Check sheet for the modelled part. Datum: model origin and axes. Units: mm. Face numbers are marked on the shaded views. A direction names the side the tool comes from. Round coordinates to 2 decimals unless told otherwise and drop trailing zeros. Order: outer loops, then holes, each group sorted by start corner. A loop starts at its lowest first (then second) coordinate and runs counter-clockwise, first axis right, second up.
(1) Depth check by flat-ended pin: pin 1 (2 mm diameter, centred on x = 0.5, y = 15.5, fed in from -Z); pin 2 (2 mm diameter, centred on y = 14, z = -48.5, fed in from +X); pin 3 (8 mm diameter, centred on x = 8.5, z = -13, fed in from +Y). Enter the tip coordinate at first touch or a pass-through.
(2) Mould release check, pull along X, two halves, no side actions. Record for the marked faces 3, 4, 5 and 6: released by +X, released by -X, zero draft, split by the parting line, or undercut.
(3) Sectioned sample at A-A, the plane x = 46.5. Enter the section's corners in (y, z).
(4) Sectioned sample at B-B, the plane y = 18.5. Enter the section's corners in (x, z).
(5) Tool access check on the marked faces 1 and 2. Record the directions out of +Z, -Z, +X, -X, +Y, -Y that give a thin tool (end or side, any length) a straight path to the whole face; none if there is none.
(6) Thickness scan on probe 1 along Z at (x, y) = (55, 10.25); probe 2 along X at (y, z) = (17.25, -13); probe 3 along X at (y, z) = (1, -40.5). Record the ranges inside material, lowest first.
(7) Sectioned sample at C-C, the plane z = -11. Enter the section's corners in (x, y).
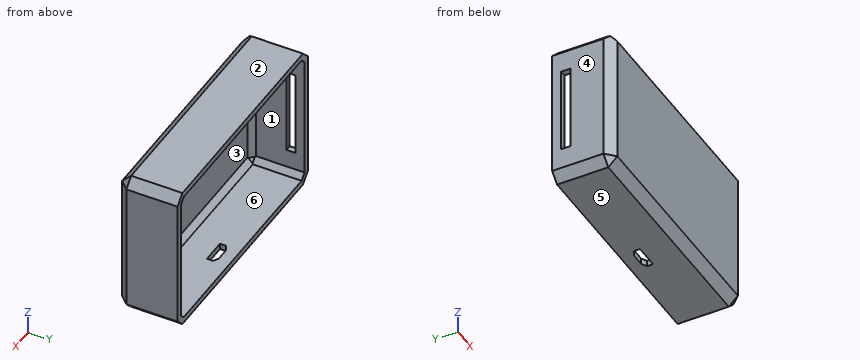
Autodesk Inventor part; units mm, degrees
ref_plane "YZ Plane" through (0, 0, 0) normal (1, 0, 0) x (0, 1, 0)
ref_plane "XZ Plane" through (0, 0, 0) normal (0, 1, 0) x (-1, 0, 0)
ref_plane "XY Plane" through (0, 0, 0) normal (0, 0, 1) x (1, 0, 0)
sketch "Náčrt1" plane through (0, 0, 0) normal (0, 1, 0) x (-1, 0, 0)
  line L0 (0, 0) -> (-80, 0)
  line L1 (-80, 0) -> (-80, -49)
  line L2 (-80, -49) -> (0, -49)
  line L3 (0, -49) -> (0, 0)
  dimension "d0" = 80
  dimension "d1" = 49
extrude "Vysunutí1" add sketch "Náčrt1" along normal blind 20
chamfer "Zkosení1" distance 3 angle 45 7 edges at (80, 10, 0) (40, 0, 0) (0, 0, -24.5) (0, 10, -49) (80, 10, -49) (40, 0, -49) (80, 0, -24.5)
chamfer "Zkosení2" distance 3 angle 45 1 edges at (0, 11.5, 0)
shell "Skořepina1" thickness 2 removed faces 1 at (27.6667, 20, -32.6667)
sketch "Náčrt2" plane through (0, 3, -46) normal (-1, 0, 0) x (0, 0, 1)
  line L0 (7, 14) -> (36, 14)
  line L1 (36, 14) -> (36, 11)
  line L2 (36, 11) -> (7, 11)
  line L3 (7, 11) -> (7, 14)
  line L4 (0, 0) -> (0, 17)
  line L5 (0, -3) -> (43, -3)
  line L6 (43, 0) -> (0, 0)
  line L7 (0, 17) -> (43, 17)
  point P0 (46, -3)
  dimension "d11" = 29
  dimension "d12" = 3
  dimension "d13" = 7
  dimension "d17" = 3
extrude "Vysunutí2" cut sketch "Náčrt2" against normal blind 2.5
sketch "Náčrt3" plane through (0, 14, -39) normal (0, 0, 1) x (1, 0, 0)
  point P0 (0, -14)
sketch "Náčrt4" plane through (77, 3, -49) normal (0, 0, -1) x (-1, 0, 0)
  line L0 (28, 13) -> (36, 13)
  line L1 (36, 13) -> (36, 10)
  line L2 (36, 10) -> (28, 10)
  line L3 (28, 10) -> (28, 13)
  line L4 (0, 0) -> (0, 17)
  line L5 (74, 0) -> (0, 0)
  line L6 (0, 17) -> (74, 17)
  point P0 (77, -3)
  dimension "d20" = 8
  dimension "d21" = 3
  dimension "d22" = 28
  dimension "d39" = 4
extrude "Vysunutí3" cut sketch "Náčrt4" against normal blind 2.5
chamfer "Zkosení3" distance 1 angle 60 1 edges at (49, 16, -48) measured on face at (49, 14, -48.3333)
chamfer "Zkosení4" distance 1 angle 60 1 edges at (41, 16, -48) measured on face at (41, 15, -48.3333)
sketch "Náčrt5" plane through (77, 3, 0) normal (0, 0, 1) x (1, 0, 0)
  point P0 (-77, -3)
sketch "Náčrt6" plane through (77, 3, -49) normal (0, 0, -1) x (-1, 0, 0)
  point P0 (77, -3)
sketch "Náčrt7" plane through (2, 3.8284, -3.8284) normal (1, 0, 0) x (0, 0, -1)
  point P0 (-3.8284, -3.8284)
properties part number "Base"
Derived:
1. pin 1: stops at z = -47.5
1. pin 2: stops at x = 78.5
1. pin 3: stops at y = 2
2. face 3: undercut
2. face 4: released by -X
2. face 5: zero draft
2. face 6: undercut
3. outline: (0, -46) - (3, -49) - (13, -49) - (13, -47) - (3.83, -47) - (2, -45.17) - (2, -3.83) - (3.83, -2) - (20, -2) - (20, 0) - (3, 0) - (0, -3) - close; (16, -49) - (20, -49) - (20, -47) - (16, -47) - close
4. outline: (0, -46) - (3, -49) - (77, -49) - (80, -46) - (80, -3) - (77, 0) - (3, 0) - (0, -3) - close; hole (2, -45.17) - (3.83, -47) - (76.17, -47) - (78, -45.17) - (78, -3.83) - (76.17, -2) - (3.83, -2) - (2, -3.83) - close
5. face 1: +Y
5. face 2: +Z, +X, -X, +Y, -Y
6. probe 1: z = -49 to -47, -2 to 0
6. probe 2: x = 0 to 2, 78 to 80
6. probe 3: x = 2 to 78
7. outline: (0, 3) - (3, 0) - (77, 0) - (80, 3) - (80, 20) - (78, 20) - (78, 3.83) - (76.17, 2) - (3.83, 2) - (2, 3.83) - (2, 14) - (0, 14) - close; (0, 17) - (2, 17) - (2, 20) - (0, 20) - close
